from build123d import *

# Parameters (mm, degrees)
SKETCH_R     = 5
PAD_DEPTH    = 20
SKETCH001_R  = 1.85
POCKET_DEPTH = 9
SKETCH002_R  = 3.65
PAD001_DEPTH = 6
FILLET_R     = 1.5


with BuildPart() as part:
    # Sketch → Pad (new body)
    with BuildSketch(Plane.XY):
        Circle(SKETCH_R)
    extrude(amount=PAD_DEPTH)

    # Sketch001 (on Face3 of Pad) → Pocket (cut)
    with BuildSketch(Plane.XY.offset(20)):
        Circle(SKETCH001_R)
    extrude(amount=-POCKET_DEPTH, mode=Mode.SUBTRACT)

    # Sketch002 (on Face2 of Pocket) → Pad001 (join)
    with BuildSketch(Plane(origin=(0, 0, 0), x_dir=(1, 0, 0), z_dir=(0, 0, -1))):
        Circle(SKETCH002_R)
    extrude(amount=PAD001_DEPTH)

    # Fillet
    fillet_edges = [part.edges().sort_by_distance(p)[0] for p in [
        (-3.65, 0, -6),
    ]]
    fillet(fillet_edges, radius=FILLET_R)


solid = part.part
Can you work these out from the model? Positions are in its coordinate system, mm. A direction names the side the tool comes from. Round coordinates to 2 decimals unless told otherwise and drop trailing zeros. Order: outer loops, then holes, each group sorted by start corner. A loop starts at its lowest first (then second) coordinate and runs counter-clockwise, first axis right, second up. Notation, with made-up numbers: (-11.5, -40) -> (42.5, -40) arc R23 ccw to (42.5, -13) -> close; hole circle Ø8 at (8, 87.5). An arc over 180 degrees is marked (long way). Write each question's results on one line, items separated by ' | '. Start each with the question number.
Item 1: If we section it at C-C, the plane z = 12.5: Write out the boundary of the cut face in (x, y).
Item 2: If we section it at A-A, the plane y = 0: Write out the boundary of the cut face in (x, z), then the cut area to 3 significant figures.
Item 3: Will these pins go through, and if not, where does the flat tip stop? pin 1 (3 mm diameter, centred on x = -3.5, z = 14.5, fed in from -Y); pin 2 (1.8 mm diameter, centred on x = 0, y = -0.5, fed in from +Z); pin 3 (5 mm diameter, centred on x = 3.5, z = 1, fed in from -Y).
Item 4: Please list where these lines run through material, in increasing order: L1, parallel to Y at x = 0, z = 14; L2, parallel to Z at x = 0.5, y = 1; L3, parallel to Z at x = -0.5, y = -4.5.
Item 5: If we section it at D-D, the plane z = -3.5: Write out the boundary of the cut face in (x, y).
Item 6: Which directions (+Z, -Z, +X, -X, +Y, -Y) give clear straight access to the entire face, cutting with the end or side of a thin tool? Please do faces 1 (the cylindrical face through (-0.401, -1.806, 15.563)), 2 (the flat face through (0, -4, 0)), 3 (the flat face through (-0.1, -2.2, 20)).
Results:
1) outline: circle Ø10 at (0, 0); hole circle Ø3.7 at (0, 0)
2) outline: (-5, 0) -> (-3.65, 0) -> (-3.65, -4.5) arc R1.5 ccw to (-2.15, -6) -> (2.15, -6) arc R1.5 ccw to (3.65, -4.5) -> (3.65, 0) -> (5, 0) -> (5, 20) -> (1.85, 20) -> (1.85, 11) -> (-1.85, 11) -> (-1.85, 20) -> (-5, 20) -> close | area: 210 mm2
3) pin 1: stops at y = -4.58 | pin 2: stops at z = 11 | pin 3: stops at y = -4.9
4) L1: y = -5 to -1.85, 1.85 to 5 | L2: z = -6 to 11 | L3: z = 0 to 20
5) outline: circle Ø7.3 at (0, 0)
6) face 1: +Z | face 2: -Z | face 3: +Z, +X, -X, +Y, -Y
